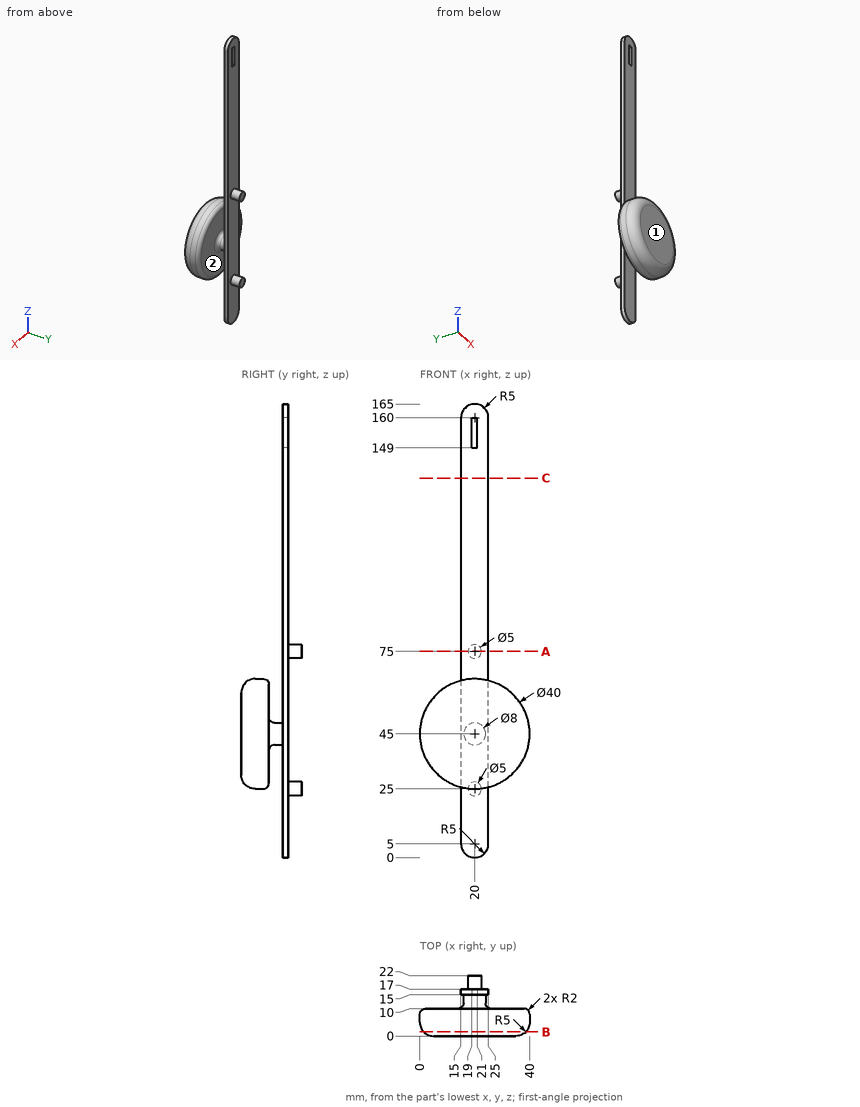
Geometry check sheet. Reference: drawing and pictorial views, mm from the part's lowest x, y, z. Round coordinates to 2 decimals unless told otherwise and drop trailing zeros. Loops run counter-clockwise (first coordinate to the right, second up) from the corner with the lowest first, then second, coordinate; pieces in that order, holes last. Notation, with made-up numbers: (-2.5, 20.5) -> (49.5, 20.5) arc R35 ccw to (49.5, 56.5) -> close; hole circle Ø3 at (-16, 67). An arc over 180 degrees is marked (long way). Use a Markdown table: item, result.
(1) Mould release check, pull along Y, two halves, no side actions. Record for the marked faces 1 and 2: released by +Y, released by -Y, zero draft, split by the parting line, or undercut.
Calculated:
| item | result |
|---|---|
| face 1 | released by -Y |
| face 2 | undercut |
(2) Sectioned sample at C-C (z = 138). Enter the section's corners in (x, y).
Calculated:
| item | result |
|---|---|
| outline | (15, 15) -> (25, 15) -> (25, 17) -> (15, 17) -> close |
(3) Sectioned sample at B-B (y = 1.5). Enter the section's corners in (x, z).
Calculated:
| item | result |
|---|---|
| outline | circle Ø37.14 at (20, 45) |
(4) Scan lines: probe 1 along Y at (x, z) = (18.5, 154); probe 2 along Z at (x, y) = (35, 9.25); probe 3 along X at (y, z) = (15.25, 54.5). Record each from-to range of solid material in increasing order.
Calculated:
| item | result |
|---|---|
| probe 1 | 15 to 17 |
| probe 2 | 32.44 to 57.56 |
| probe 3 | 15 to 25 |
(5) Sectioned sample at A-A (z = 75). Enter the section's corners in (x, y).
Calculated:
| item | result |
|---|---|
| outline | (15, 15) -> (25, 15) -> (25, 17) -> (22.5, 17) -> (22.5, 22) -> (17.5, 22) -> (17.5, 17) -> (15, 17) -> close |
(6) Go/stop test with flat-tipped pins: P1, Ø1.5, axis at y = 17.5, z = 96.5, coming from the +X side; P2, Ø0.6, axis at x = 19.5, y = 16.5, coming from the +Z side; P3, Ø1, axis at y = 16, z = 153, coming from the -X side. Record where each tip stops, or that it passes through.
Calculated:
| item | result |
|---|---|
| P1 | x = 25 |
| P2 | z = 165 |
| P3 | x = 15 |
